Verification items for the finished model (mm, model axes). Round coordinates to 2 decimals unless told otherwise and drop trailing zeros. Order: outer loops, then holes, each group sorted by start corner. A loop starts at its lowest first (then second) coordinate and runs counter-clockwise, first axis right, second up. Notation, with made-up numbers: (83.5, 28.25) -> (132.5, 28.25) arc R26 ccw to (132.5, 47.25) -> close; hole circle Ø1 at (-13.5, -28). An arc over 180 degrees is marked (long way). Answer in a Markdown table with one row per item. Add a question column.
```python
from build123d import *

# Parameters (mm, degrees)
SKETCH1_R             = 3
BOSS_EXTRUDE1_DEPTH   = 2
SKETCH6_R             = 3
BOSS_EXTRUDE2_DEPTH   = 2
BOSS_EXTRUDE2_2_DEPTH = 2
SKETCH7_R             = 1.5
SKETCH7_R_2           = 6.85
CUT_EXTRUDE4_DEPTH    = 10
SKETCH8_R             = 2
CUT_EXTRUDE5_DEPTH    = 175.152232257
SKETCH9_R             = 2.5
CUT_EXTRUDE6_DEPTH    = 10
CUT_EXTRUDE7_DEPTH    = 10
FILLET1_R             = 5


with BuildPart() as part:
    # Sketch1 → Boss-Extrude1 (new body)
    with BuildSketch(Plane.XY):
        Polygon((-135, -20.635083269), (-135, -50), (135, -50), (135, -20.635083269), (135, 40), (135, 50), (-135, 50), (-135, 40), align=None)
        with Locations((-127, -46)):
            Circle(SKETCH1_R, mode=Mode.SUBTRACT)
        with Locations((-120, 46)):
            Circle(SKETCH1_R, mode=Mode.SUBTRACT)
        with Locations(Location((120, 46, 0), (0, 0, 180))):
            Circle(SKETCH1_R, mode=Mode.SUBTRACT)
        with Locations(Location((127, -46, 0), (0, 0, 180))):
            Circle(SKETCH1_R, mode=Mode.SUBTRACT)
        Polygon((-126, 40), (-97, 40), (-97, 25), (-79, 25), (-79, -25), (-97, -25), (-97, -40), (-126, -40), align=None, mode=Mode.SUBTRACT)
        Polygon((-70, -31.5), (-42, -31.5), (-42, -21.5), (-4, -21.5), (4, -21.5), (42, -21.5), (42, -31.5), (70, -31.5), (70, 31.5), (42, 31.5), (42, 21.5), (4, 21.5), (-4, 21.5), (-42, 21.5), (-42, 31.5), (-70, 31.5), align=None, mode=Mode.SUBTRACT)
        Polygon((97, -40), (126, -40), (126, 40), (97, 40), (97, 25), (79, 25), (79, -25), (97, -25), align=None, mode=Mode.SUBTRACT)
    extrude(amount=BOSS_EXTRUDE1_DEPTH)


with BuildPart() as body_2:
    # Sketch6 → Boss-Extrude2 (new body)
    with BuildSketch(Plane.XY.offset(2)):
        Polygon((75, 110), (135, 110), (135, 50), (-135, 50), (-135, 110), align=None)
        with Locations((-125, 94)):
            Circle(SKETCH6_R, mode=Mode.SUBTRACT)
        with Locations((125, 94)):
            Circle(SKETCH6_R, mode=Mode.SUBTRACT)
    extrude(amount=-BOSS_EXTRUDE2_DEPTH)

    # Combine1: union part
    add(part.part)


with BuildPart() as body_3:
    # Sketch6 → Boss-Extrude2 2 (new body)
    with BuildSketch(Plane.XY.offset(2)):
        with BuildLine():
            Line((-135, -50), (135, -50))
            Line((135, -50), (135, -55))
            ThreePointArc((135, -55), (133.535533906, -58.535533906), (130, -60))
            Line((130, -60), (-130, -60))
            ThreePointArc((-130, -60), (-133.535533906, -58.535533906), (-135, -55))
            Line((-135, -55), (-135, -50))
        make_face()
    extrude(amount=-BOSS_EXTRUDE2_2_DEPTH)


with BuildPart() as body_2_1:
    add(body_2.part)

    # Combine2: union body 3
    add(body_3.part)

    # Sketch7 → Cut-Extrude4 (cut)
    with BuildSketch(Plane.XY.offset(2)):
        with Locations((11.25, -49.495190528)):
            Circle(SKETCH7_R)
        with Locations((-11.25, -49.495190528)):
            Circle(SKETCH7_R)
        with Locations((0, -30.009618943)):
            Circle(SKETCH7_R)
        with Locations((90.234667928, 98.180240786)):
            Circle(SKETCH7_R)
        with Locations((0, -43)):
            Circle(SKETCH7_R_2)
        with Locations((112.734667928, 98.180240786)):
            Circle(SKETCH7_R)
        with Locations((101.484667928, 78.6946692)):
            Circle(SKETCH7_R)
        with Locations((101.484667928, 91.685050257)):
            Circle(SKETCH7_R_2)
        with Locations((-101.484667928, 91.685050257)):
            Circle(SKETCH7_R_2)
        with Locations(Location((-101.484667928, 78.6946692, 0), (0, 0, 180))):
            Circle(SKETCH7_R)
        with Locations((-112.734667928, 98.180240786)):
            Circle(SKETCH7_R)
        with Locations((-90.234667928, 98.180240786)):
            Circle(SKETCH7_R)
    extrude(amount=-CUT_EXTRUDE4_DEPTH, mode=Mode.SUBTRACT)

    # Sketch8 → Cut-Extrude5 (cut, through all)
    with BuildSketch(Plane(origin=(0, 0, 0), x_dir=(-1, 0, 0), z_dir=(0, 0, -1))):
        with Locations((-130, -15)):
            Circle(SKETCH8_R)
        with Locations((-130, 15)):
            Circle(SKETCH8_R)
        with Locations((-75, -15)):
            Circle(SKETCH8_R)
        with Locations((-75, 15)):
            Circle(SKETCH8_R)
        with Locations((75, -15)):
            Circle(SKETCH8_R)
        with Locations((75, 15)):
            Circle(SKETCH8_R)
        with Locations((130, -15)):
            Circle(SKETCH8_R)
        with Locations((130, 15)):
            Circle(SKETCH8_R)
    extrude(amount=-CUT_EXTRUDE5_DEPTH, mode=Mode.SUBTRACT)

    # Sketch9 → Cut-Extrude6 (cut)
    with BuildSketch(Plane(origin=(0, 0, 0), x_dir=(-1, 0, 0), z_dir=(0, 0, -1))):
        with Locations((81.5, 93.898069018)):
            Circle(SKETCH9_R)
        with Locations((81.5, 63.898069018)):
            Circle(SKETCH9_R)
        with Locations((-81.5, 93.898069018)):
            Circle(SKETCH9_R)
        with Locations((-81.5, 63.898069018)):
            Circle(SKETCH9_R)
    extrude(amount=-CUT_EXTRUDE6_DEPTH, mode=Mode.SUBTRACT)

    # Sketch10 → Cut-Extrude7 (cut)
    with BuildSketch(Plane.XY.offset(2)):
        with BuildLine():
            Line((-130, -60), (130, -60))
            ThreePointArc((130, -60), (133.535533906, -58.535533906), (135, -55))
            Line((135, -55), (-135, -55))
            ThreePointArc((-135, -55), (-133.535533906, -58.535533906), (-130, -60))
        make_face()
    extrude(amount=-CUT_EXTRUDE7_DEPTH, mode=Mode.SUBTRACT)

    # Fillet1
    fillet1_edges = [body_2_1.edges().sort_by_distance(p)[0] for p in [
        (135, -55, 1),
        (-135, -55, 1),
    ]]
    fillet(fillet1_edges, radius=FILLET1_R)


solid = body_2_1.part
```
1) Cross-section at B-B, the plane z = 1. Give the number of separate pieces and of enclosed holes in the cut face, and give its area (3 significant figures).
2) Draft check along X on faces 1 (the face through (134, -53, 1)), 2 (the face through (2, 47, 0)), 3 (the face through (117.14, 45.1, 0.99)). Enter one of: +X half, -X half, draft (parallel to the pull), parting line (faces both ways), or undercut.
3) Depth check by flat-ended pin: P1, Ø1.8, axis at x = 112.73, y = 98.18, coming from the +Z side. Enter the tip coordinate at first touch or a pass-through.
4) Thickness scan on L1, parallel to X at y = 18, z = 1.25; L2, parallel to Y at x = -75, z = 1.55; L3, parallel to Y at x = 120, z = 0.6. Record the ranges inside material, lowest first. Write a range as [from, to].
5) Cross-section at A-A, the plane y = 46. Record the boundary of the cut face in (x, z), and give its area (3 significant figures).
Results below:
| question | item | result |
|---|---|---|
| 1 | separate pieces | 1 |
| 1 | enclosed holes | 33 |
| 1 | area | 30,100 mm² |
| 2 | face 1 | +X half |
| 2 | face 2 | draft |
| 2 | face 3 | undercut |
| 3 | P1 | through |
| 4 | L1 | [-135, -126], [-79, -70], [70, 79], [126, 135] |
| 4 | L2 | [-55, -17], [-13, 13], [17, 110] |
| 4 | L3 | [-55, -40], [40, 43], [49, 110] |
| 5 | outline | (-135, 0) -> (-123, 0) -> (-123, 2) -> (-135, 2) -> close; (-117, 0) -> (117, 0) -> (117, 2) -> (-117, 2) -> close; (123, 0) -> (135, 0) -> (135, 2) -> (123, 2) -> close |
| 5 | area | 516 mm² |
